Autodesk Inventor part; units mm, degrees
ref_plane "YZ Plane" through (0, 0, 0) normal (1, 0, 0) x (0, 1, 0)
ref_plane "XZ Plane" through (0, 0, 0) normal (0, 1, 0) x (-1, 0, 0)
ref_plane "XY Plane" through (0, 0, 0) normal (0, 0, 1) x (1, 0, 0)
sketch "Sketch1" plane through (0, 0, 0) normal (1, 0, 0) x (0, 1, 0)
  line L0 (0, 0) -> (18.2735, 0) construction
  line L1 (18.2735, 0) -> (18.8146, -20.5646) construction
  line L2 (22.3653, -155.5) -> (0, -155.5)
  line L3 (0, -155.5) -> (0, 0)
  line L4 (0, -186.6) -> (0, 31.1)
  line L5 (22.1995, -149.2) -> (0, -149.2) construction
  line L6 (-4.4731, 0) -> (26.8383, 0) construction
  line L7 (0, 0) -> (16.0387, -2.3398)
  line L8 (17.75, -4.3188) -> (17.75, -19.5)
  line L9 (17.75, -19.5) -> (18.8146, -20.5646)
  line L10 (18.8146, -20.5646) -> (22.3653, -155.5)
  arc A0 (17.75, -4.3188) -> (16.0387, -2.3398) centre (15.75, -4.3188) ccw
  dimension "d0" = 155.5
  dimension "d1" = 36.547
  dimension "d2" = 44.399
  dimension "d3" = 149.2
  dimension "d4" = 19.5
  dimension "d5" = 35.5
  dimension "d6" = 45
  dimension "d7" = 8.3
  dimension "d8" = 2
revolve "Revolution1" add sketch "Sketch1" angle 360 about axis through (0, 0, -155.5) along (0, 0, 1)
chamfer "Chamfer1" distance 3 angle 45 1 edges at (0, -22.3653, -155.5)
sketch "Sketch3" plane through (0, 0, 0) normal (0, 1, 0) x (-1, 0, 0)
  line L0 (7.95, 0) -> (7.95, -19.5)
  arc A0 (7.95, -19.5) -> (19.5695, -30.4825) centre (18.95, -19.5) ccw
  line L1 (19.5695, -30.4825) -> (19.5695, 0)
  line L2 (19.5695, 0) -> (7.95, 0)
  line L3 (0, -186.6) -> (0, 31.1)
  line L4 (31.8888, 0) -> (-31.3156, 0)
  point P0 (0, 0)
  dimension "d19" = 15.9
  dimension "d20" = 30.5
  dimension "d21" = 11
extrude "Extrusion2" cut sketch "Sketch3" along normal through all both and the other way through all
mirror "Mirror2" about plane through (0, 0, 0) normal (1, 0, 0) of "Extrusion2"
properties material "Steel, Alloy"
Can you work these out from the model? Positions are in its coordinate system, mm. A direction names the side the tool comes from. Give positions to 0.01 mm unless a question says otherwise; leave off trailing zeros. Order: outer loops, then holes, each group sorted by start corner. A loop starts at its lowest first (then second) coordinate and runs counter-clockwise, first axis right, second up. Notation, with made-up numbers: (-29.75, 84) - (24.25, 84) arc R24 ccw to (24.25, 97) - close; hole circle Ø5 at (80, -30). An arc over 180 degrees is marked (long way). Use a Markdown table: item, result. Add a question column.
Q1. On a 3-axis mill with a long thin cutter (end or side, diameter ignored), from which of +Z, -Z, +X, -X, +Y, -Y can I reach the whole of each face in a straight line? I mean faces 1 (the flat face through (7.95, 0, -10)), 2 (the conical face through (0.905, -20.555, -87.456)), 3 (the flat face through (-7.95, 0, -10)), 4 (the cylindrical face through (-0.12, 17.75, -12.02)). Say none if no direction works.
Q2. If we section it at D-D on z = -27.5: Write out the boundary of the cut face in (x, y), plus the area to 3 significant figures.
Q3. If we section it at A-A on z = -10.5: Write out the boundary of the cut face in (x, y).
Q4. I'm going to push flat-ended pins straight in: pin 1 (3 mm diameter, centred on x = -3.5, y = 16, fed in from +Z); pin 2 (3 mm diameter, centred on x = 6.5, z = -81.5, fed in from -Y); pin 3 (4 mm diameter, centred on x = -14.5, z = -67.5, fed in from +Y). Where does each tip first touch, or does it pass through?
Q5. If we section it at C-C on z = -79: Write out the boundary of the cut face in (x, y), plus the area to 3 significant figures.
Q6. Please list where these lines run through material, in increasing order: line 1 along Y through (x, z) = (12.5, -108); line 2 along Y through (x, z) = (16.5, -89); line 3 along X through (y, z) = (9, -56.5).
Q7. If we section it at B-B on z = -49: Write out the boundary of the cut face in (x, y).
Answers follow:
| question | item | result |
|---|---|---|
| 1 | face 1 | +Z, +X, +Y, -Y |
| 1 | face 2 | +Z |
| 1 | face 3 | +Z, -X, +Y, -Y |
| 1 | face 4 | +Z, +Y |
| 2 | outline | (-11.4, -15.2) arc R19 ccw to (11.4, -15.2) - (11.4, 15.2) arc R19 ccw to (-11.4, 15.2) - close |
| 2 | area | 811 mm^2 |
| 3 | outline | (-7.95, -15.87) arc R17.75 ccw to (7.95, -15.87) - (7.95, 15.87) arc R17.75 ccw to (-7.95, 15.87) - close |
| 4 | pin 1 | stops at z = -2.17 |
| 4 | pin 2 | stops at y = -19.8 |
| 4 | pin 3 | stops at y = 15.68 |
| 5 | outline | circle Ø40.7 at (0, 0) |
| 5 | area | 1,300 mm^2 |
| 6 | line 1 | y = -17.02 to 17.02 |
| 6 | line 2 | y = -12.36 to 12.36 |
| 6 | line 3 | x = -17.59 to 17.59 |
| 7 | outline | circle Ø39.13 at (0, 0) |
